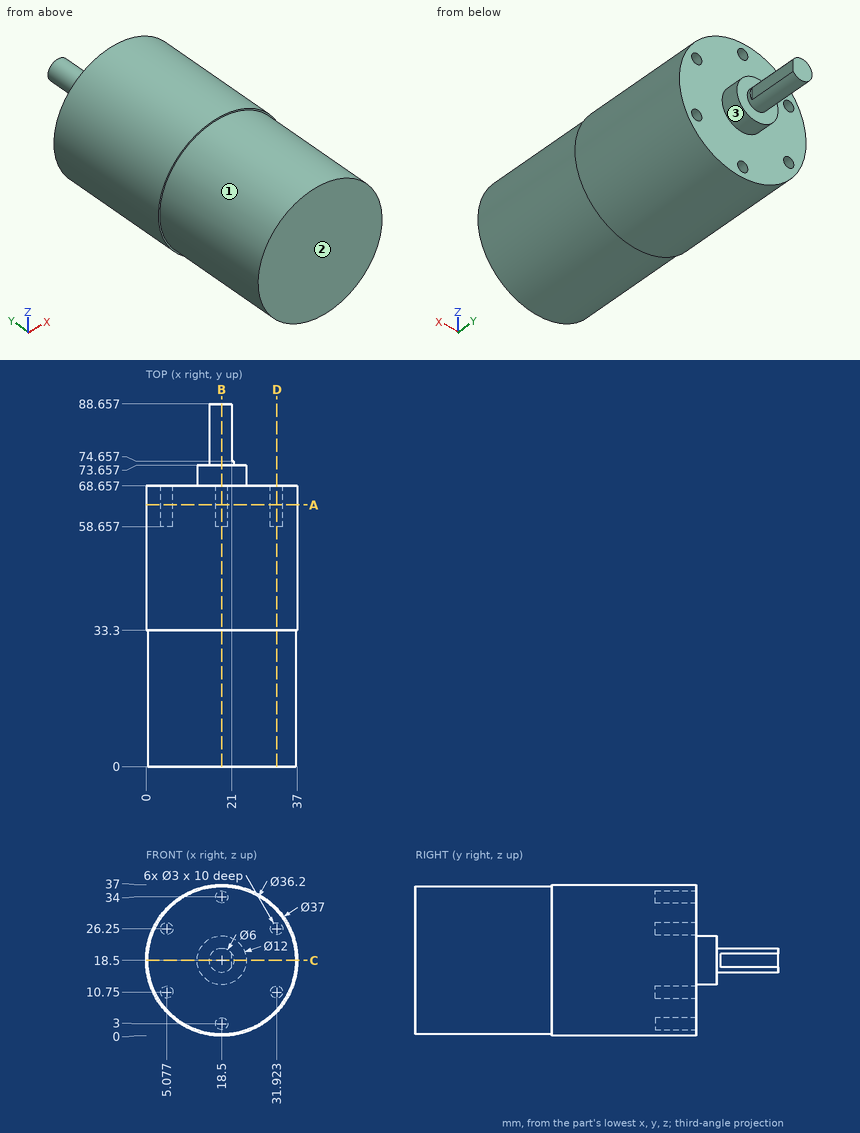
Study the drawing (mm; zero at the part's minimum x, y, z) and answer. A direction names the side the tool comes from. Coordinates: 2 decimals unless noted, no trailing zeros. Write each loop counter-clockwise with the first axis right and the second up, starting at its lowest first coordinate (ties: lowest second). Pieces come first, ordered by that corner, then holes. Notation, with made-up numbers: M -12,-40 L 25,-40 A28 ccw 25,-19 Z; hole C 64.5,-22.5 d10. An arc over 180 degrees is marked long. Use a Markdown table: item, result. Add a question column.
1. Given P1, Ø3.5, axis at x = 31.92, z = 10.75, coming from the +Y side; P2, Ø11, axis at x = 22.5, z = 10.5, coming from the +Y side; P3, Ø2, axis at y = 62.5, z = 16, coming from the +X side, each flat-ended and moving along its own axis, determine where each tip first touches the part or whether it passes through.
2. Section D-D (x = 32) is taken. Give the vertices of the cut face in (y, z).
3. Section A-A (y = 64) is taken. Count the separate pieces of the cut face and the enclosed holes in it, plus the area to 3 significant figures.
4. Section B-B (x = 18.5) is taken. Give the vertices of the cut face in (y, z), plus the area to 3 significant figures.
5. Straight lines are drawn through the part: line 1 along X through (y, z) = (64.5, 26.25); line 2 along Z through (x, y) = (19, 67) (1 decimal); line 3 along Y through (x, z) = (11, 20). For each, find the intervals that lie inside material, in ascending order. Write a range as [from, to].
6. Which of the six approach directions +Z, -Z, +X, -X, +Y, -Y give full straight-line access (tool end or side, diameter ignored) to the marked faces 1, 2 and 3?
7. Section C-C (z = 18.5) is taken. Give the vertices of the cut face in (x, y).
Data:
| question | item | result |
|---|---|---|
| 1 | P1 | stops at y = 68.66 |
| 1 | P2 | stops at y = 73.66 |
| 1 | P3 | stops at x = 36.94 |
| 2 | outline | M 0,6.44 L 33.3,6.44 L 33.3,5.85 L 68.66,5.85 L 68.66,9.25 L 58.66,9.25 L 58.66,12.25 L 68.66,12.25 L 68.66,24.75 L 58.66,24.75 L 58.66,27.75 L 68.66,27.75 L 68.66,31.15 L 33.3,31.15 L 33.3,30.56 L 0,30.56 Z |
| 3 | separate pieces | 1 |
| 3 | enclosed holes | 6 |
| 3 | area | 1,030 mm2 |
| 4 | outline | M 0,0.4 L 33.3,0.4 L 33.3,0 L 68.66,0 L 68.66,1.5 L 58.66,1.5 L 58.66,4.5 L 68.66,4.5 L 68.66,12.5 L 73.66,12.5 L 73.66,15.5 L 88.66,15.5 L 88.66,21.5 L 73.66,21.5 L 73.66,24.5 L 68.66,24.5 L 68.66,32.5 L 58.66,32.5 L 58.66,35.5 L 68.66,35.5 L 68.66,37 L 33.3,37 L 33.3,36.6 L 0,36.6 Z |
| 4 | area | 2,600 mm2 |
| 5 | line 1 | x = [1.7, 3.58], [6.58, 30.42], [33.42, 35.3] |
| 5 | line 2 | z = [0, 1.6], [4.4, 32.6], [35.4, 37] |
| 5 | line 3 | y = [0, 68.66] |
| 6 | face 1 | -Y |
| 6 | face 2 | +Z, -Z, +X, -X, -Y |
| 6 | face 3 | +Y |
| 7 | outline | M 0,33.3 L 0.4,33.3 L 0.4,0 L 36.6,0 L 36.6,33.3 L 37,33.3 L 37,68.66 L 24.5,68.66 L 24.5,73.66 L 21.5,73.66 L 21.5,74.66 L 21,74.66 L 21,88.66 L 15.5,88.66 L 15.5,73.66 L 12.5,73.66 L 12.5,68.66 L 0,68.66 Z |
